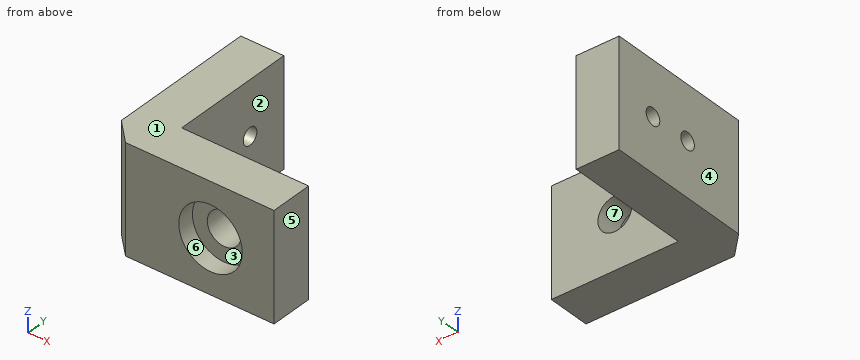
from build123d import *

# Parameters (mm, degrees)
F1_DEPTH       = 12.7
F3_D           = 4
F3_DEPTH       = 12.7
F3_CBORE_D     = 7.5
F3_CBORE_DEPTH = 2
F4_SIZE        = 2.54
F6_D           = 2


with BuildPart() as f1:
    # F0 (on Top) → F1 (new body)
    with BuildSketch(Plane.XY):
        Polygon((10.949644, 17.412821), (5.869644, 17.412821), (5.869644, -2.667179), (25.949644, -2.667179), (25.949644, 2.412821), (10.949644, 2.412821), align=None)
    extrude(amount=F1_DEPTH)

    # F3
    with Locations(Plane.XZ.offset(2.667179)):
        with Locations((18.449644, 6.35)):
            CounterBoreHole(F3_D / 2, F3_CBORE_D / 2, F3_CBORE_DEPTH, depth=F3_DEPTH)

    # F4
    f4_edges = [f1.edges().sort_by_distance(p)[0] for p in [
        (5.869644, -2.667179, 6.35),
    ]]
    chamfer(f4_edges, length=F4_SIZE)

    # F6 (through all)
    with Locations(Plane(origin=(5.869644, 0, 0), x_dir=(0, -1, 0), z_dir=(-1, 0, 0))):
        with Locations((-7.372821, 6.35), (-12.452821, 6.35)):
            Hole(F6_D / 2)


solid = f1.part
Read the model definition and answer for the solid it produces. Units are mm, in the model's axes. Face numbers are marked on the shaded views. A direction names the side the tool comes from. Coordinates: 2 decimals unless noted, no trailing zeros. Loops run counter-clockwise (first coordinate to the right, second up) from the corner with the lowest first, then second, coordinate; pieces in that order, holes last. Notation, with made-up numbers: (19, 84.25) -> (26, 84.25) arc R23 ccw to (26, 100.25) -> close; hole circle Ø2 at (11.5, -7). An arc over 180 degrees is marked (long way). Write item = value, one per line. Start each with the question number.
1) The mould has two halves that part along X. Classify the marked faces 4, 5, 6 and 7: pulls with the +X half, pulls with the -X half, needs draft (parallel to the pull), parting line crosses it, or undercut.
2) The part is cut by section B-B, the plane x = 9.75. Determine the outline of the cut face in (y, z).
3) Find the intervals of material crossed by L1, parallel to Y at x = 9.5, z = 6.75; L2, parallel to X at y = 6.5, z = 7; L3, parallel to Y at x = 15.5, z = 11.5, in increasing order. Write a range as from..to.
4) For the marked faces 1, 2 and 3, determine the directions among +Z, -Z, +X, -X, +Y, -Y from which every point of the face is accessible in a straight line to the end or side of a thin tool.
5) The part is cut by section A-A, the plane z = 6.35. Determine the outline of the cut face in (x, y), plus the area to 3 significant figures.
6) Given P1, Ø4, axis at x = 19.5, z = 5, coming from the -Y side; P2, Ø6, axis at x = 10, y = 9.5, coming from the -Z side; P3, Ø6, axis at y = 8.5, z = 3, coming from the +X side; P4, Ø6.5, axis at x = 19, z = 5, coming from the +Y side, each flat-ended and moving along its own axis, determine where each tip first touches the part or whether it passes through.
7) The part is cut by section C-C, the plane z = 10.5. Determine the outline of the cut face in (x, y), plus the area to 3 significant figures.
8) The part is cut by section D-D, the plane x = 19.25. Determine the outline of the cut face in (y, z), plus the area to 3 significant figures.
Result:
q1.face_4 = pulls with the -X half
q1.face_5 = pulls with the +X half
q1.face_6 = undercut
q1.face_7 = undercut
q2.outline = (-2.67, 0) -> (17.41, 0) -> (17.41, 12.7) -> (-2.67, 12.7) -> close; hole circle Ø2 at (7.37, 6.35); hole circle Ø2 at (12.45, 6.35)
q3.L1 = -2.67..6.46, 8.29..11.54, 13.37..17.41
q3.L2 = 5.87..10.95
q3.L3 = -2.67..2.41
q4.face_1 = +Z, +X, -X, +Y, -Y
q4.face_2 = +Z, -Z, +X, +Y
q4.face_3 = -Y
q5.outline = (5.87, -0.13) -> (8.41, -2.67) -> (14.7, -2.67) -> (14.7, -0.67) -> (16.45, -0.67) -> (16.45, 2.41) -> (10.95, 2.41) -> (10.95, 6.37) -> (5.87, 6.37) -> close; (5.87, 8.37) -> (10.95, 8.37) -> (10.95, 11.45) -> (5.87, 11.45) -> close; (5.87, 13.45) -> (10.95, 13.45) -> (10.95, 17.41) -> (5.87, 17.41) -> close; (20.45, -0.67) -> (22.2, -0.67) -> (22.2, -2.67) -> (25.95, -2.67) -> (25.95, 2.41) -> (20.45, 2.41) -> close
q5.area = 127 mm²
q6.P1 = -0.67
q6.P2 = 0
q6.P3 = 10.95
q6.P4 = 2.41
q7.outline = (5.87, -0.13) -> (8.41, -2.67) -> (25.95, -2.67) -> (25.95, 2.41) -> (10.95, 2.41) -> (10.95, 17.41) -> (5.87, 17.41) -> close
q7.area = 175 mm²
q8.outline = (-2.67, 0) -> (2.41, 0) -> (2.41, 4.52) -> (-0.67, 4.52) -> (-0.67, 2.69) -> (-2.67, 2.69) -> close; (-2.67, 10.01) -> (-0.67, 10.01) -> (-0.67, 8.18) -> (2.41, 8.18) -> (2.41, 12.7) -> (-2.67, 12.7) -> close
q8.area = 38.6 mm²
